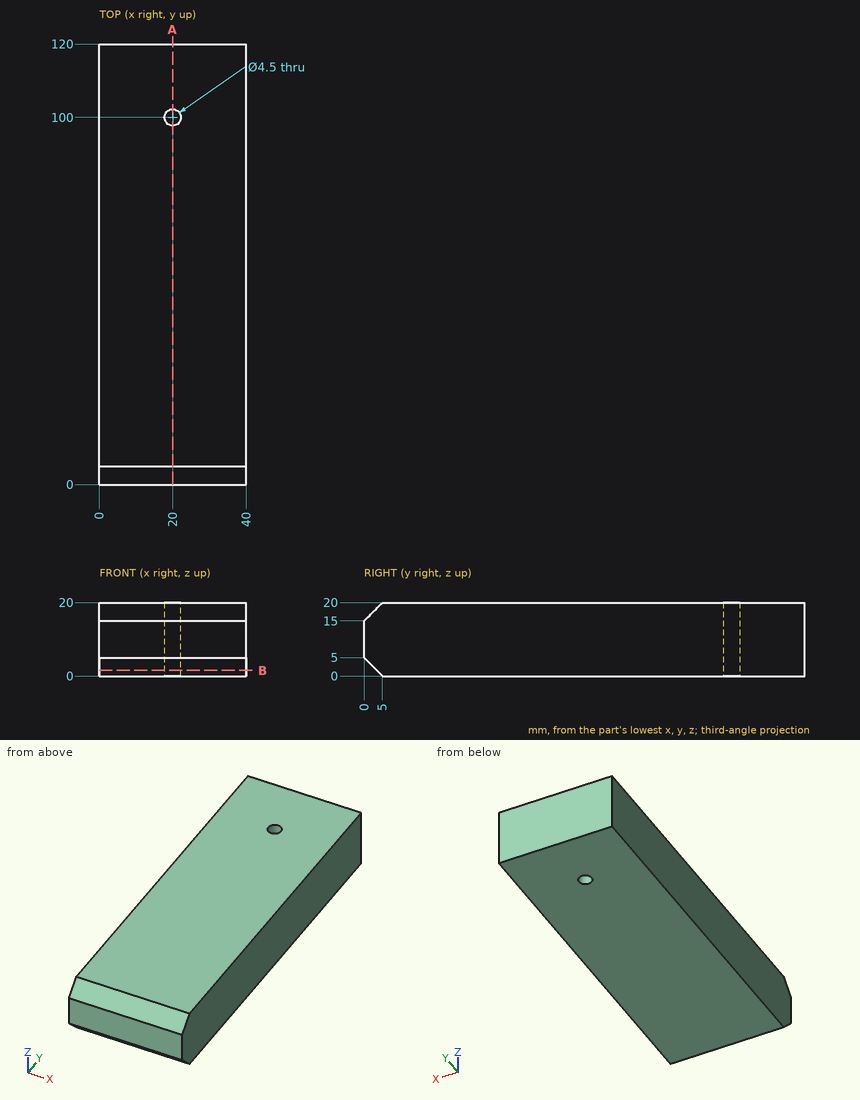
Geometry check sheet. Reference: drawing and pictorial views, mm from the part's lowest x, y, z. Give positions to 0.01 mm unless a question says otherwise; leave off trailing zeros. Loops run counter-clockwise (first coordinate to the right, second up) from the corner with the lowest first, then second, coordinate; pieces in that order, holes last. Notation, with made-up numbers: (-10, 72.5) -> (9, 72.5) arc R22 cw to (9, 96.5) -> close; hole circle Ø9 at (19.5, 40). An arc over 180 degrees is marked (long way). Answer in a Markdown table with one row per item. Add a question column.
1) Cross-section at A-A on x = 20. Record the boundary of the cut face in (y, z).
2) Material ranges on probe 1 along X at (y, z) = (100, 14.5); probe 2 along Y at (x, z) = (20, 12.75); probe 3 along Y at (x, z) = (20, 4.25), recorded low to high. Write a range as from..to.
3) Cross-section at B-B on z = 1.5. Record the boundary of the cut face in (x, y), and give its area (3 significant figures).
Outcome:
| question | item | result |
|---|---|---|
| 1 | outline | (0, 5) -> (5, 0) -> (97.75, 0) -> (97.75, 20) -> (5, 20) -> (0, 15) -> close; (102.25, 0) -> (120, 0) -> (120, 20) -> (102.25, 20) -> close |
| 2 | probe 1 | x = 0..17.75, 22.25..40 |
| 2 | probe 2 | y = 0..97.75, 102.25..120 |
| 2 | probe 3 | y = 0.75..97.75, 102.25..120 |
| 3 | outline | (0, 3.5) -> (40, 3.5) -> (40, 120) -> (0, 120) -> close; hole circle Ø4.5 at (20, 100) |
| 3 | area | 4,640 mm^2 |
